```python
from build123d import *

# Parameters (mm, degrees)
SKETCH_1_R          = 1.55
EXTRUDE_1_DEPTH     = 5
SKETCH_2_R          = 1.55
CUT_EXTRUDE_1_DEPTH = 5
FILLET_1_R          = 10
SKETCH_4_R          = 0.8
SKETCH_4_W          = 23
SKETCH_4_H          = 13
SKETCH_4_R_2        = 1.55
CUT_EXTRUDE_2_DEPTH = 5
EXTRUDE_START       = 5
SKETCH_5_R          = 3.05
SKETCH_5_R_2        = 1.55
SKETCH_5_R_3        = 3
EXTRUDE_2_DEPTH     = 5
SKETCH_8_R          = 1.55
CUT_EXTRUDE_4_DEPTH = 11
SKETCH_6_R          = 1.6
CUT_EXTRUDE_6_DEPTH = 10
CHAMFER_1_SIZE      = 0.3
FILLET_2_R          = 7


with BuildPart() as part:
    # 草图1 → 凸台-拉伸1 (new body)
    with BuildSketch(Plane(origin=(0, 0, 0), x_dir=(1, 0, 0), z_dir=(0, 1, 0))):
        Polygon((-11, 30), (-25, 15), (-25, -15), (25, -15), (25, 15), (11, 30), align=None)
        with Locations(Location((-11.75, 5, 0), (0, 0, 270))):
            Circle(SKETCH_1_R, mode=Mode.SUBTRACT)
        with Locations(Location((11.75, 5, 0), (0, 0, 90))):
            Circle(SKETCH_1_R, mode=Mode.SUBTRACT)
    extrude(amount=EXTRUDE_1_DEPTH)

    # 草图2 → 切除-拉伸1 (cut)
    with BuildSketch(Plane(origin=(0, 5, 0), x_dir=(1, 0, 0), z_dir=(0, 1, 0))):
        with Locations(Location((-4.5, 26, 0), (0, 0, 270))):
            Circle(SKETCH_2_R)
        with Locations(Location((4.5, 26, 0), (0, 0, 90))):
            Circle(SKETCH_2_R)
    extrude(amount=-CUT_EXTRUDE_1_DEPTH, mode=Mode.SUBTRACT)

    # 圆角1
    fillet_1_edges = [part.edges().sort_by_distance(p)[0] for p in [
        (-25, 2.5, -15),
        (-11, 2.5, -30),
        (11, 2.5, -30),
        (25, 2.5, -15),
    ]]
    fillet(fillet_1_edges, radius=FILLET_1_R)

    # 草图4 → 切除-拉伸2 (cut)
    # profile 1 of 3: a face of its own
    with BuildSketch(Plane.XZ):
        with Locations(Location((19.75, -5, 0), (0, 0, 270))):
            Circle(SKETCH_4_R)
    # profile 2 of 3: a face of its own
    with BuildSketch(Plane.XZ):
        with Locations(Location((-7.25, -5, 0), (0, 0, 90))):
            Circle(SKETCH_4_R)
    # profile 3 of 3: a face of its own
    with BuildSketch(Plane.XZ):
        with Locations((6.25, -5)):
            Rectangle(SKETCH_4_W, SKETCH_4_H)
        with Locations((11.75, -5)):
            Circle(SKETCH_4_R_2, mode=Mode.SUBTRACT)
    extrude(amount=-CUT_EXTRUDE_2_DEPTH, mode=Mode.SUBTRACT)

    # 草图5 → 凸台-拉伸2 (add)
    # profile 1 of 3: a face of its own
    with BuildSketch(Plane(origin=(0, 5, 0), x_dir=(1, 0, 0), z_dir=(0, 1, 0)).offset(EXTRUDE_START)):
        with Locations(Location((-4.5, 26, 0), (0, 0, 270))):
            Circle(SKETCH_5_R)
        with Locations(Location((-4.5, 26, 0), (0, 0, 270))):
            Circle(SKETCH_5_R_2, mode=Mode.SUBTRACT)
    # profile 2 of 3: a face of its own
    with BuildSketch(Plane(origin=(0, 5, 0), x_dir=(1, 0, 0), z_dir=(0, 1, 0)).offset(EXTRUDE_START)):
        with Locations(Location((4.5, 26, 0), (0, 0, 270))):
            Circle(SKETCH_5_R)
        with Locations(Location((4.5, 26, 0), (0, 0, 270))):
            Circle(SKETCH_5_R_2, mode=Mode.SUBTRACT)
    # profile 3 of 3: a face of its own
    with BuildSketch(Plane(origin=(0, 5, 0), x_dir=(1, 0, 0), z_dir=(0, 1, 0)).offset(EXTRUDE_START)):
        with Locations(Location((-11.75, 5, 0), (0, 0, 270))):
            Circle(SKETCH_5_R_3)
    extrude(amount=-EXTRUDE_2_DEPTH)

    # 草图8 → 切除-拉伸4 (cut)
    with BuildSketch(Plane.XZ):
        with Locations(Location((-11.75, -5, 0), (0, 0, 90))):
            Circle(SKETCH_8_R)
    extrude(amount=-CUT_EXTRUDE_4_DEPTH, mode=Mode.SUBTRACT)

    # 草图6 → 切除-拉伸6 (cut)
    with BuildSketch(Plane(origin=(0, 5, 0), x_dir=(1, 0, 0), z_dir=(0, 1, 0))):
        with Locations(Location((-9, -11.5, 0), (0, 0, 270))):
            Circle(SKETCH_6_R)
        with Locations(Location((9, -11.5, 0), (0, 0, 270))):
            Circle(SKETCH_6_R)
    extrude(amount=-CUT_EXTRUDE_6_DEPTH, mode=Mode.SUBTRACT)

    # 倒角1
    chamfer_1_edges = [part.edges().sort_by_distance(p)[0] for p in [
        (-9, 0, 9.9),
        (9, 0, 9.9),
    ]]
    chamfer(chamfer_1_edges, length=CHAMFER_1_SIZE)

    # 圆角2
    fillet_2_edges = [part.edges().sort_by_distance(p)[0] for p in [
        (25, 2.5, 15),
        (-25, 2.5, 15),
    ]]
    fillet(fillet_2_edges, radius=FILLET_2_R)


solid = part.part
```
Source: CAD feature listing. Evaluate the final solid. Frame: model axes, mm. A direction names the side the tool comes from. Round coordinates to 2 decimals unless told otherwise and drop trailing zeros. Write each loop counter-clockwise with the first axis right and the second up, starting at its lowest first coordinate (ties: lowest second). Pieces come first, ordered by that corner, then holes. Notation, with made-up numbers: M 58.25,65 L 65.25,65 A19 ccw 65.25,71 Z; hole C 89,39.5 d1. An arc over 180 degrees is marked long. Answer as a JSON object with one key per item and string values. Group by question number.
(1) Ray query, line 1 (X direction, y = 3.9, z = -5); line 2 (X direction, y = 7, z = -26); line 3 (X direction, y = 2.75, z = 0.5). Return the intervals inside material, ascending. Write a range as [from, to].
(2) Mould query, pull axis Z, two halves, no side actions, for faces 4 (the flat face through (0, 2, 15)), 5 (the flat face through (-5.25, 2, -5)), 6 (the cylindrical face through (-7.79, 2.46, -5.59)), 7 (the cylindrical face through (-24.284, 2.535, -14.774)). Classes: +Z half, -Z half, draft (parallel to the pull), parting line (faces both ways), or undercut.
(3) Reachability of faces 1 (the flat face through (6, 2, 1.5)), 2 (the cylindrical face through (-10.85, 7.54, -2.14)), 3 (the cylindrical face through (24.284, 2.535, -14.774)) from +Z, -Z, +X, -X, +Y, -Y: full face, straight path, thin tool, end or side. Return the list, or none.
(4) Section query D-D on y = 3.5. State how many separate pieces and enclosed holes the cut face has, then the cut area to 3 significant figures.
(5) Section query C-C on y = 7.5. Output: boundary loops of the cut face in (x, z), then the cut area to 3 significant figures.
(6) Section query A-A on x = 0. Output: boundary loops of the cut face in (y, z), then the cut area to 3 significant figures.
(7) First-contact query: pin 1 (2.5 mm diameter, centred on x = -7.25, z = -5, fed in from +Y); pin 2 (3.5 mm diameter, centred on x = -9, z = 11.5, fed in from -Y); pin 3 (3 mm diameter, centred on x = 4.5, z = -26, fed in from +Y); pin 4 (6 mm diameter, centred on x = -19, y = 1.5, fed in from -Z). Flat tips, straight axial feed; report the tip coordinate or a pass-through.
(8) Section query B-B on z = -5. Output: boundary loops of the cut face in (x, y), then the cut area to 3 significant figures.
Computed values:
{
 "1": {"line 1": "[-25, -13.3], [-10.2, -8.05], [-6.45, -5.25], [17.75, 18.95], [20.55, 25]", "line 2": "[-7.55, -6.05], [-2.95, -1.45], [1.45, 2.95], [6.05, 7.55]", "line 3": "[-25, -5.25], [17.75, 25]"},
 "2": {"face 4": "+Z half", "face 5": "undercut", "face 6": "undercut", "face 7": "-Z half"},
 "3": {"face 1": "+Y, -Y", "face 2": "+Y", "face 3": "-Z, +X, +Y, -Y"},
 "4": {"separate pieces": "1", "enclosed holes": "8", "area": "1,670 mm^2"},
 "5": {"outline": "C -11.75,-5 d6; C -4.5,-26 d6.1; C 4.5,-26 d6.1; hole C -11.75,-5 d3.1; hole C -4.5,-26 d3.1; hole C 4.5,-26 d3.1", "area": "64.1 mm^2"},
 "6": {"outline": "M 0,-30 L 5,-30 L 5,-11.5 L 0,-11.5 Z; M 0,1.5 L 5,1.5 L 5,15 L 0,15 Z", "area": "160 mm^2"},
 "7": {"pin 1": "y = 5", "pin 2": "y = 0.15", "pin 3": "through", "pin 4": "z = -24.64"},
 "8": {"outline": "M -25,0 L -13.3,0 L -13.3,10 L -14.75,10 L -14.75,5 L -25,5 Z; M -10.2,0 L -8.05,0 L -8.05,5 L -8.75,5 L -8.75,10 L -10.2,10 Z; M -6.45,0 L -5.25,0 L -5.25,5 L -6.45,5 Z; M 17.75,0 L 18.95,0 L 18.95,5 L 17.75,5 Z; M 20.55,0 L 25,0 L 25,5 L 20.55,5 Z", "area": "118 mm^2"}
}
